from build123d import *

# Parameters (mm, degrees)
BOSS_EXTRUDE1_DEPTH = 3.175
HOLE1_OUTLINE_R     = 1.7
HOLE1_DEPTH         = 3.175


# Read off the part's stored shape, not the designer's step: Hole1
with BuildPart() as part:
    # Sketch1 → Boss-Extrude1 (new body)
    with BuildSketch(Plane(origin=(0, 0, 0), x_dir=(1, 0, 0), z_dir=(0, 1, 0))):
        Polygon((-0.009590706, 15.307381957), (-12.509590706, -6.343253138), (12.490409294, -6.343253138), align=None)
    extrude(amount=BOSS_EXTRUDE1_DEPTH)

    # Hole1 outline → Hole1 (cut)
    with BuildSketch(Plane(origin=(0, 0, 0), x_dir=(1, 0, 0), z_dir=(0, 1, 0))):
        with Locations((8.221235052, -3.912057057)):
            Circle(HOLE1_OUTLINE_R)
        with Locations((-8.228764373, -3.907710002)):
            Circle(HOLE1_OUTLINE_R)
        with Locations((0, 10.336233865)):
            Circle(HOLE1_OUTLINE_R)
    extrude(amount=HOLE1_DEPTH, mode=Mode.SUBTRACT)


solid = part.part
The listing builds one solid part. Answer for the finished solid, in the listing's coordinates (mm). Give positions to 0.01 mm unless a question says otherwise; leave off trailing zeros. Loops run counter-clockwise (first coordinate to the right, second up) from the corner with the lowest first, then second, coordinate; pieces in that order, holes last. Notation, with made-up numbers: (17.5, -37.5) - (45.5, -37.5) arc R31 ccw to (45.5, -0.5) - close; hole circle Ø6 at (4.5, 27.25). An arc over 180 degrees is marked (long way). Use one line per item in the form item = value.
1. Section B-B on y = 2.35 is taken. Give the vertices of the cut face in (x, z).
Calculated:
outline = (-12.51, 6.34) - (-0.01, -15.31) - (12.49, 6.34) - close; hole circle Ø3.4 at (-8.23, 3.91); hole circle Ø3.4 at (0, -10.34); hole circle Ø3.4 at (8.22, 3.91)
2. Find the intervals of material crossed by line 1 along X through (y, z) = (1.15, 4.75); line 2 along Z through (x, y) = (8, 2.6); line 3 along Z through (x, y) = (-9.25, 0.8), in increasing order. Write a range as [from, to].
Calculated:
line_1 = [-11.59, -9.71], [-6.75, 6.74], [9.7, 11.57]
line_2 = [-1.43, 2.23], [5.6, 6.34]
line_3 = [0.7, 2.55], [5.27, 6.34]
3. Section C-C on x = 9.25 is taken. Give the vertices of the cut face in (y, z) (3 decimals).
Calculated:
outline = (0, 0.731) - (3.175, 0.731) - (3.175, 2.559) - (0, 2.559) - close; (0, 5.265) - (3.175, 5.265) - (3.175, 6.343) - (0, 6.343) - close
4. Section A-A on x = -1 is taken. Give the vertices of the cut face in (y, z) (3 decimals).
Calculated:
outline = (0, -13.592) - (3.175, -13.592) - (3.175, -11.711) - (0, -11.711) - close; (0, -8.961) - (3.175, -8.961) - (3.175, 6.343) - (0, 6.343) - close
5. The mould has two halves that part along Z. Classify faces 1 (the face through (-6.66, 1.57, 4.56)), 2 (the face through (0, 3.175, -2)), 3 (the face through (-6.172, 1.565, -4.634)): pulls with the +Z half, pulls with the -Z half, needs draft (parallel to the pull), parting line crosses it, or undercut.
Calculated:
face_1 = undercut
face_2 = needs draft
face_3 = pulls with the -Z half
6. Section D-D on z = -8 is taken. Give the vertices of the cut face in (x, y) (1 decimal), then the cut area to 3 significant figures.
Calculated:
outline = (-4.2, 0) - (4.2, 0) - (4.2, 3.2) - (-4.2, 3.2) - close
area = 26.8 mm^2
